```python
from build123d import *

# Parameters (mm, degrees)
ESQUISSE1_R                  = 0.5
BASE_EXTRUSION_DEPTH         = 1
ESQUISSE2_R                  = 3.75
BOSS_EXTRU_1_DEPTH           = 0.5
ESQUISSE3_R                  = 3.75
BOSS_EXTRU_2_DEPTH           = 2.5
ESQUISSE4_R                  = 3.25
ENL_V_MAT_EXTRU_1_DEPTH      = 1.5
ESQUISSE5_R                  = 1.5
ENL_V_MAT_EXTRU_2_DEPTH      = 4.5
ESQUISSE7_R                  = 2.2
ENL_V_MAT_EXTRU_4_DEPTH      = 3
DENTS_DEPTH                  = 3
R_P_TITION_CIRCULAIRE1_COUNT = 24


with BuildPart() as part:
    # Esquisse1 → Base-Extrusion (new body, symmetric)
    with BuildSketch(Plane.XY):
        with BuildLine():
            Line((1.488676655, 10.683961455), (2.260839574, 4.435364907))
            ThreePointArc((2.260839574, 4.435364907), (2.974200379, 2.974200379), (4.435364907, 2.260839574))
            Line((4.435364907, 2.260839574), (10.683961455, 1.488676655))
            ThreePointArc((10.683961455, 1.488676655), (12, 0), (10.683961455, -1.488676655))
            Line((10.683961455, -1.488676655), (4.435364907, -2.260839574))
            ThreePointArc((4.435364907, -2.260839574), (2.974200379, -2.974200379), (2.260839574, -4.435364907))
            Line((2.260839574, -4.435364907), (1.488676655, -10.683961455))
            ThreePointArc((1.488676655, -10.683961455), (0, -12), (-1.488676655, -10.683961455))
            Line((-1.488676655, -10.683961455), (-2.260839574, -4.435364907))
            ThreePointArc((-2.260839574, -4.435364907), (-2.974200379, -2.974200379), (-4.435364907, -2.260839574))
            Line((-4.435364907, -2.260839574), (-10.683961455, -1.488676655))
            ThreePointArc((-10.683961455, -1.488676655), (-12, 0), (-10.683961455, 1.488676655))
            Line((-10.683961455, 1.488676655), (-4.435364907, 2.260839574))
            ThreePointArc((-4.435364907, 2.260839574), (-2.974200379, 2.974200379), (-2.260839574, 4.435364907))
            Line((-2.260839574, 4.435364907), (-1.488676655, 10.683961455))
            ThreePointArc((-1.488676655, 10.683961455), (0, 12), (1.488676655, 10.683961455))
        make_face()
        with Locations((10.5, 0)):
            Circle(ESQUISSE1_R, mode=Mode.SUBTRACT)
        with Locations((8.5, 0)):
            Circle(ESQUISSE1_R, mode=Mode.SUBTRACT)
        with Locations((6.5, 0)):
            Circle(ESQUISSE1_R, mode=Mode.SUBTRACT)
        with Locations((0, -10.5)):
            Circle(ESQUISSE1_R, mode=Mode.SUBTRACT)
        with Locations((0, -8.5)):
            Circle(ESQUISSE1_R, mode=Mode.SUBTRACT)
        with Locations((0, -6.5)):
            Circle(ESQUISSE1_R, mode=Mode.SUBTRACT)
        with Locations((0, 10.5)):
            Circle(ESQUISSE1_R, mode=Mode.SUBTRACT)
        with Locations((0, 8.5)):
            Circle(ESQUISSE1_R, mode=Mode.SUBTRACT)
        with Locations((0, 6.5)):
            Circle(ESQUISSE1_R, mode=Mode.SUBTRACT)
        with Locations((-10.5, 0)):
            Circle(ESQUISSE1_R, mode=Mode.SUBTRACT)
        with Locations((-8.5, 0)):
            Circle(ESQUISSE1_R, mode=Mode.SUBTRACT)
        with Locations((-6.5, 0)):
            Circle(ESQUISSE1_R, mode=Mode.SUBTRACT)
    extrude(amount=BASE_EXTRUSION_DEPTH, both=True)

    # Esquisse2 → Boss.-Extru.1 (add)
    with BuildSketch(Plane.XY.offset(1)):
        Circle(ESQUISSE2_R)
    extrude(amount=BOSS_EXTRU_1_DEPTH)

    # Esquisse3 → Boss.-Extru.2 (add)
    with BuildSketch(Plane(origin=(0, 0, -1), x_dir=(-1, 0, 0), z_dir=(0, 0, -1))):
        Circle(ESQUISSE3_R)
    extrude(amount=BOSS_EXTRU_2_DEPTH)

    # Esquisse4 → Enlèv. mat.-Extru.1 (cut)
    with BuildSketch(Plane.XY.offset(1.5)):
        Circle(ESQUISSE4_R)
    extrude(amount=-ENL_V_MAT_EXTRU_1_DEPTH, mode=Mode.SUBTRACT)

    # Esquisse5 → Enlèv. mat.-Extru.2 (cut, through all)
    with BuildSketch(Plane.XY):
        Circle(ESQUISSE5_R)
    extrude(amount=-ENL_V_MAT_EXTRU_2_DEPTH, mode=Mode.SUBTRACT)

    # Esquisse7 → Enlèv. mat.-Extru.4 (cut)
    with BuildSketch(Plane(origin=(0, 0, -3.5), x_dir=(-1, 0, 0), z_dir=(0, 0, -1))):
        Circle(ESQUISSE7_R)
    extrude(amount=-ENL_V_MAT_EXTRU_4_DEPTH, mode=Mode.SUBTRACT)

    # Esquisse6 → Dents (cut)
    with BuildSketch(Plane(origin=(0, 0, -3.5), x_dir=(-1, 0, 0), z_dir=(0, 0, -1))):
        with BuildLine():
            Line((0, 2.8), (0.288653169, 2.180981281))
            ThreePointArc((0.288653169, 2.180981281), (0, 2.2), (-0.288653169, 2.180981281))
            Line((-0.288653169, 2.180981281), (0, 2.8))
        make_face()
    dents = extrude(amount=-DENTS_DEPTH, mode=Mode.SUBTRACT)

    # Répétition circulaire1: Dents ×24 about axis
    r_p_tition_circulaire1_axis = Axis((0, 0, 0), (0, 0, 1))
    for i in range(1, R_P_TITION_CIRCULAIRE1_COUNT):
        add(dents.rotate(r_p_tition_circulaire1_axis, i * 360 / R_P_TITION_CIRCULAIRE1_COUNT), mode=Mode.SUBTRACT)


solid = part.part
```
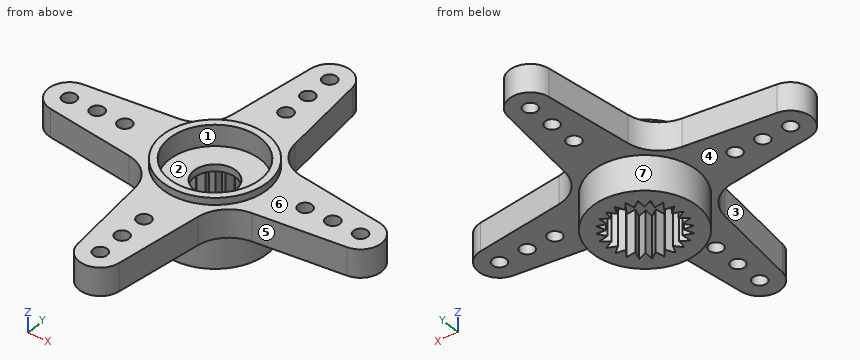
Design review of the part built by this model. Coordinates are the model's own, in mm. Face numbers are marked on the shaded views. A direction names the side the tool comes from. Give positions to 0.01 mm unless a question says otherwise; leave off trailing zeros. Order: outer loops, then holes, each group sorted by start corner. A loop starts at its lowest first (then second) coordinate and runs counter-clockwise, first axis right, second up. Notation, with made-up numbers: (17.25, -21) - (41.25, -21) arc R10 ccw to (41.25, -9) - close; hole circle Ø5 at (-31, 75.5). An arc over 180 degrees is marked (long way). Use a Markdown table: item, result. Add a question column.
(1) Add section A-A on x = -8.5. Give the boundary of the cut face in (y, z), then the cut area to 3 significant figures.
(2) Clearance check with a flat-ended pin moving along its axis: P1, Ø4, axis at x = 4.5, y = 4, coming from the +Z side. State where the tip first meets the part, or that it passes through.
(3) Wall thickness on probe 1 along X at (y, z) = (-2.5, -1.85); probe 2 along X at (y, z) = (2.5, 0.65); probe 3 along Z at (x, y) = (-0.5, -1.5): over which ranges is each line inside the solid? List them lowest first. Write a range as [from, to].
(4) Add section C-C on x = 5.5. Give the boundary of the cut face in (y, z), then the cut area to 3 significant figures.
(5) Machinability: for the marked faces 5, 6 and 7, which of the approach directions +Z, -Z, +X, -X, +Y, -Y give a long, thin tool a straight path to every point of the face, cutting with its end or side? Answer none if there is none.
(6) Mouldability with a two-part tool opening along Y and no side actions: class the marked faces 1, 2, 3 and 4 as +Y half, -Y half, draft (parallel to the pull), parting line (faces both ways), or undercut.
(7) Add section B-B on y = -6.5. Give the boundary of the cut face in (x, z).
Report:
| question | item | result |
|---|---|---|
| 1 | outline | (-1.76, -1) - (-0.5, -1) - (-0.5, 1) - (-1.76, 1) - close; (0.5, -1) - (1.76, -1) - (1.76, 1) - (0.5, 1) - close |
| 1 | area | 5.03 mm² |
| 2 | P1 | stops at z = 1 |
| 3 | probe 1 | x = [-2.8, -0.76], [-0.55, -0.14], [0.14, 0.55], [0.76, 2.8] |
| 3 | probe 2 | x = [-3.64, -2.08], [2.08, 3.64] |
| 3 | probe 3 | z = [-0.5, 0] |
| 4 | outline | (-2.13, -1) - (2.13, -1) - (2.13, 1) - (-2.13, 1) - close |
| 4 | area | 8.52 mm² |
| 5 | face 5 | +Z, -Z, +X, -Y |
| 5 | face 6 | +Z |
| 5 | face 7 | -Z |
| 6 | face 1 | undercut |
| 6 | face 2 | undercut |
| 6 | face 3 | -Y half |
| 6 | face 4 | draft |
| 7 | outline | (-2.01, -1) - (-0.5, -1) - (-0.5, 1) - (-2.01, 1) - close; (0.5, -1) - (2.01, -1) - (2.01, 1) - (0.5, 1) - close |
